Design review of the part built by this model. Coordinates are the model's own, in mm. Face numbers are marked on the shaded views. A direction names the side the tool comes from. Round coordinates to 2 decimals unless told otherwise and drop trailing zeros. Order: outer loops, then holes, each group sorted by start corner. A loop starts at its lowest first (then second) coordinate and runs counter-clockwise, first axis right, second up.
from build123d import *

# Parameters (mm, degrees)
SKETCH2_R                = 1.455
BOSS_EXTRUDE3_DEPTH      = 6
SKETCH3_R                = 2.5
BOSS_EXTRUDE4_DEPTH      = 3
CUT_EXTRUDE1_DEPTH       = 10.669539803
CUT_EXTRUDE1_DEPTH_BACK  = 10.669539803
SKETCH4_R                = 0.5
SKETCH6_R                = 1.575
BOSS_EXTRUDE5_DEPTH      = 0.15
CUT_EXTRUDE3_START       = -3
CUT_EXTRUDE3_OUTLINE_R   = 2.5
CUT_EXTRUDE3_OUTLINE_R_2 = 1.455
CUT_EXTRUDE3_DEPTH       = 3
CUT_EXTRUDE4_START       = -1
SKETCH10_R               = 1.455
CUT_EXTRUDE4_DEPTH       = 1
FILLET1_R                = 0.25
SKETCH11_R               = 1.455
SKETCH11_R_2             = 1.355
CUT_EXTRUDE5_DEPTH       = 1.5


# Read off the part's stored shape, not the designer's step: Cut-Extrude3
with BuildPart() as part:
    # Sketch2 → Boss-Extrude3 (new body)
    with BuildSketch(Plane(origin=(0, 0, 0), x_dir=(0, 0, -1), z_dir=(1, 0, 0))):
        Circle(SKETCH2_R)
    extrude(amount=BOSS_EXTRUDE3_DEPTH)

    # Sketch3 → Boss-Extrude4 (add)
    with BuildSketch(Plane(origin=(6, 0, 0), x_dir=(0, 0, -1), z_dir=(1, 0, 0))):
        Circle(SKETCH3_R)
    extrude(amount=BOSS_EXTRUDE4_DEPTH)

    # Sketch4 → Cut-Extrude1 (cut, two sides: drawn at the far end of the back side and taken through both)
    with BuildSketch(Plane(origin=(0, 0, 0), x_dir=(1, 0, 0), z_dir=(0, 1, 0)).offset(-CUT_EXTRUDE1_DEPTH_BACK)):
        with Locations(Location((1, 0, 0), (0, 0, 270))):
            Circle(SKETCH4_R)
    extrude(amount=CUT_EXTRUDE1_DEPTH + CUT_EXTRUDE1_DEPTH_BACK, mode=Mode.SUBTRACT)

    # Sketch6 → Boss-Extrude5 (add)
    with BuildSketch(Plane.YZ.offset(1)):
        with Locations(Location((0, 0, 0), (0, 0, 270))):
            Circle(SKETCH6_R)
    extrude(amount=BOSS_EXTRUDE5_DEPTH)

    # Sketch7 → Revolve1 (revolve)
    with BuildSketch(Plane.XY, mode=Mode.PRIVATE) as revolve1_sk:
        Polygon((1.15, 1.825), (0, 0.8), (1.15, 0.8), align=None)
    revolve(revolve1_sk.sketch.rotate(Axis((9.45, 0, 0), (-1, 0, 0)), 90), axis=Axis((9.45, 0, 0), (-1, 0, 0)))

    # Cut-Extrude3 outline → Cut-Extrude3 (cut)
    with BuildSketch(Plane(origin=(9, 0, 0), x_dir=(0, 0, -1), z_dir=(1, 0, 0)).offset(CUT_EXTRUDE3_START)):
        Circle(CUT_EXTRUDE3_OUTLINE_R)
        Circle(CUT_EXTRUDE3_OUTLINE_R_2, mode=Mode.SUBTRACT)
    extrude(amount=CUT_EXTRUDE3_DEPTH, mode=Mode.SUBTRACT)

    # Sketch10 → Cut-Extrude4 (cut)
    with BuildSketch(Plane(origin=(9, 0, 0), x_dir=(0, 0, -1), z_dir=(1, 0, 0)).offset(CUT_EXTRUDE4_START)):
        with Locations(Location((0, 0, 0), (0, 0, 250.863842603))):
            Circle(SKETCH10_R)
    extrude(amount=CUT_EXTRUDE4_DEPTH, mode=Mode.SUBTRACT)

    # Fillet1
    fillet1_edges = [part.edges().sort_by_distance(p)[0] for p in [
        (8, 0, 1.455),
    ]]
    fillet(fillet1_edges, radius=FILLET1_R)

    # Sketch11 → Cut-Extrude5 (cut)
    with BuildSketch(Plane(origin=(1.15, 0, 0), x_dir=(0, 0, -1), z_dir=(1, 0, 0))):
        Circle(SKETCH11_R)
        with Locations(Location((0, 0, 0), (0, 0, 110.610126659))):
            Circle(SKETCH11_R_2, mode=Mode.SUBTRACT)
    extrude(amount=CUT_EXTRUDE5_DEPTH, mode=Mode.SUBTRACT)


solid = part.part
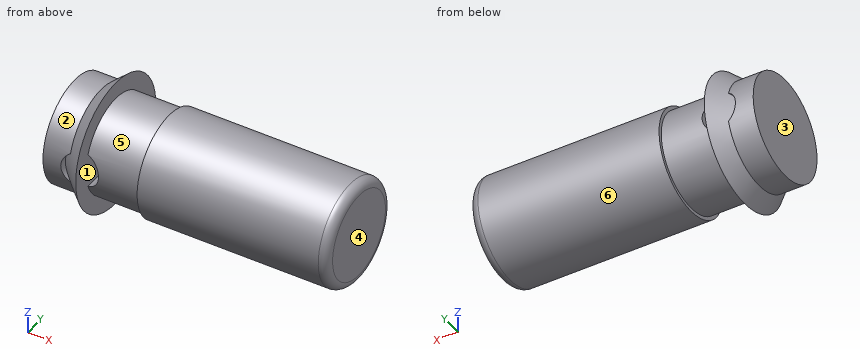
1) Take a section at D-D on x = 2. Give the boundary of the cut face in (y, z) (3 decimals).
Results:
outline: circle Ø2.71 at (0, 0)
2) Take a section at B-B on y = 0. Give the boundary of the cut face in (x, z) (3 decimals), plus the area to 3 significant figures.
Results:
outline: (0, -1.455) - (0.735, -1.455) - (1.15, -1.825) - (1.15, -1.355) - (2.65, -1.355) - (2.65, -1.455) - (7.75, -1.455) arc R0.25 ccw to (8, -1.205) - (8, 1.205) arc R0.25 ccw to (7.75, 1.455) - (2.65, 1.455) - (2.65, 1.355) - (1.15, 1.355) - (1.15, 1.825) - (0.735, 1.455) - (0, 1.455) - close; hole (1, -0.5) - (1, 0.5) arc R0.5 ccw to start; hole (1.15, -0.477) arc R0.5 ccw to (1.15, 0.477) - close
area: 22.5 mm2
3) Take a section at A-A on z = 0. Give the boundary of the cut face in (x, y) (3 decimals).
Results:
outline: (0, -1.455) - (0.5, -1.455) - (0.5, -1.246) - (1.15, -1.825) - (1.15, 1.825) - (0.5, 1.246) - (0.5, 1.455) - (0, 1.455) - close; (1.5, -1.355) - (2.65, -1.355) - (2.65, -1.455) - (7.75, -1.455) arc R0.25 ccw to (8, -1.205) - (8, 1.205) arc R0.25 ccw to (7.75, 1.455) - (2.65, 1.455) - (2.65, 1.355) - (1.5, 1.355) - close; hole (0.5, -0.8) - (1, -0.8) - (1, 0.8) - (0.5, 0.8) - close
4) The part is to be moulded in two halves that separate along X. For the marked faces 4, 5 and 6, say which applies: released by +X, released by -X, zero draft, split by the parting line, or undercut.
Results:
face 4: released by +X
face 5: undercut
face 6: zero draft
5) Clearance check with a flat-ended pin moving along its axis: P1, Ø2, axis at x = 6.5, y = 0.5, coming from the -Z side (3 decimals). State where the tip first meets the part, or that it passes through.
Results:
P1: stops at z = -1.455
6) Take a section at C-C on x = 5. Give the boundary of the cut face in (y, z) (3 decimals), plus the area to 3 significant figures.
Results:
outline: circle Ø2.91 at (0, 0)
area: 6.65 mm2
7) For the marked faces 1, 2 and 3, list the 3-axis set-ups (+Z, -Z, +X, -X, +Y, -Y) from which the entire face can be reached by the end or side of a thin tool; tool diameter is ignored.
Results:
face 1: none
face 2: -X
face 3: +Z, -Z, -X, +Y, -Y
8) To check wall thickness, follow line 1 along Z through (x, y) = (6.25, -0.75); line 2 along Z through (x, y) = (0.75, -0.55); line 3 along Z through (x, y) = (4.5, 0.05). State the ranges of each line that lie inside material, in increasing order.
Results:
line 1: z = -1.25 to 1.25
line 2: z = -1.36 to -0.43, 0.43 to 1.36
line 3: z = -1.45 to 1.45
